Work out the finished part from the listing and answer in its coordinate system (mm). A direction names the side the tool comes from. Round coordinates to 2 decimals unless told otherwise and drop trailing zeros. Write each loop counter-clockwise with the first axis right and the second up, starting at its lowest first coordinate (ties: lowest second). Pieces come first, ordered by that corner, then holes.
1. Find section B-B (x = -99.25). Write down the section's boundary in (y, z), and give its area (3 significant figures).
2. A flat-ended cylindrical pin translates along its axis: pin 1 Ø2 at (x, y) = (-101.5, 207.5) entering from +Z. Find the tip coordinate at first contact, or state that the pin passes through.
3. Determine the mould class of faces 4 (the face through (-94.494, 212, 6)), 5 (the face through (-106.266, 204.004, 5.71)), 6 (the face through (-100, 210.103, 6)), 7 (the face through (-92.494, 219, 6)) for opening direction Y: pulls with the +Y half, pulls with the -Y half, needs draft (parallel to the pull), parting line crosses it, or undercut.
4. Find section D-D (y = 218). Write down the section's boundary in (x, z).
5. A tool of negligible diameter and unlimited length cuts with its end or side. For faces 1 (the face through (-92.945, 203.981, 5.71)), 2 (the face through (-104.494, 212, 6)), 3 (the face through (-99, 224, 6.9)), from which of +Z, -Z, +X, -X, +Y, -Y can it reach the whole face along a straight path? Write none if from no direction.
6. Find section C-C (x = -103.5). Write down the section's boundary in (y, z), and give its area (3 significant figures).
7. Find section A-A (y = 212). Write down the section's boundary in (x, z), and give its area (3 significant figures).
8. Straight lines are drawn through the part: probe 1 along Y at (x, z) = (-101.25, 5.9); probe 2 along Y at (x, z) = (-99.75, 5.2); probe 3 along Z at (x, y) = (-93.25, 217.5). For each, find the intervals that lie inside material, in ascending order.
```python
from build123d import *

# Parameters (mm, degrees)
SKETCH1_W           = 14.2
SKETCH1_H           = 32.2
BOSS_EXTRUDE1_DEPTH = 1.4
SKETCH2_R           = 1
SKETCH2_W           = 10
SKETCH2_H           = 3.8
CUT_EXTRUDE1_DEPTH  = 1.4
SKETCH3_R           = 2.11
BOSS_EXTRUDE2_DEPTH = 3.2
FILLET1_R           = 1.5
SKETCH5_R           = 2.75
BOSS_EXTRUDE3_DEPTH = 0.5


with BuildPart() as part:
    # Sketch1 → Boss-Extrude1 (new body)
    with BuildSketch(Plane.XY.offset(5)):
        with Locations((-99.59415338, 219.653192448)):
            Rectangle(SKETCH1_W, SKETCH1_H)
    extrude(amount=BOSS_EXTRUDE1_DEPTH)

    # Sketch2 → Cut-Extrude1 (cut)
    with BuildSketch(Plane.XY.offset(6.4)):
        with Locations((-99.59415338, 234.253192448)):
            Circle(SKETCH2_R)
        with Locations((-99.59415338, 205.853192448)):
            Circle(SKETCH2_R)
        with Locations((-99.49415338, 212.003192448)):
            Rectangle(SKETCH2_W, SKETCH2_H)
    extrude(amount=-CUT_EXTRUDE1_DEPTH, mode=Mode.SUBTRACT)

    # Sketch3 → Boss-Extrude2 (add)
    with BuildSketch(Plane.XY.offset(6.4)):
        with Locations((-100.055672153, 226.235056066)):
            Circle(SKETCH3_R)
    extrude(amount=BOSS_EXTRUDE2_DEPTH)

    # Fillet1
    fillet1_edges = [part.edges().sort_by_distance(p)[0] for p in [
        (-106.69415338, 235.753192448, 5.7),
        (-92.49415338, 235.753192448, 5.7),
        (-92.49415338, 203.553192448, 5.7),
        (-106.69415338, 203.553192448, 5.7),
    ]]
    fillet(fillet1_edges, radius=FILLET1_R)

    # Sketch5 → Boss-Extrude3 (add)
    with BuildSketch(Plane.XY.offset(6.4)):
        with Locations((-100.056084646, 226.274312916)):
            Circle(SKETCH5_R)
    extrude(amount=BOSS_EXTRUDE3_DEPTH)


solid = part.part
```
Worked answers:
1. outline: (203.55, 5) - (204.91, 5) - (204.91, 6.4) - (203.55, 6.4) - close; (206.79, 5) - (210.1, 5) - (210.1, 6.4) - (206.79, 6.4) - close; (213.9, 5) - (233.31, 5) - (233.31, 6.4) - (228.9, 6.4) - (228.9, 6.9) - (228.19, 6.9) - (228.19, 9.6) - (224.28, 9.6) - (224.28, 6.9) - (223.65, 6.9) - (223.65, 6.4) - (213.9, 6.4) - close; (235.19, 5) - (235.75, 5) - (235.75, 6.4) - (235.19, 6.4) - close
1. area: 47.7 mm2
2. pin 1: stops at z = 6.4
3. face 4: undercut
3. face 5: pulls with the -Y half
3. face 6: undercut
3. face 7: needs draft
4. outline: (-106.69, 5) - (-92.49, 5) - (-92.49, 6.4) - (-106.69, 6.4) - close
5. face 1: +Z, -Z, +X, -Y
5. face 2: +Z, -Z
5. face 3: +Z
6. outline: (203.55, 5) - (210.1, 5) - (210.1, 6.4) - (203.55, 6.4) - close; (213.9, 5) - (235.75, 5) - (235.75, 6.4) - (213.9, 6.4) - close
6. area: 39.8 mm2
7. outline: (-106.69, 5) - (-104.49, 5) - (-104.49, 6.4) - (-106.69, 6.4) - close; (-94.49, 5) - (-92.49, 5) - (-92.49, 6.4) - (-94.49, 6.4) - close
7. area: 5.88 mm2
8. probe 1: y = 203.55 to 210.1, 213.9 to 235.75
8. probe 2: y = 203.55 to 204.87, 206.84 to 210.1, 213.9 to 233.27, 235.24 to 235.75
8. probe 3: z = 5 to 6.4
